from build123d import *

# Parameters (mm, degrees)
BOSS_EXTRUDE1_DEPTH = 155.575
SKETCH3_R           = 2.6289
CUT_EXTRUDE2_DEPTH  = 25.4
SKETCH4_R           = 2.6289
CUT_EXTRUDE3_DEPTH  = 25.4


with BuildPart() as part:
    # Sketch1 → Boss-Extrude1 (new body)
    with BuildSketch(Plane.XY):
        Polygon((3.484491601, 6.45148445), (-3.844903625, 6.243400471), (-7.329395227, -0.208083979), (-3.484491601, -6.45148445), (3.844903625, -6.243400471), (7.329395227, 0.208083979), align=None)
    extrude(amount=BOSS_EXTRUDE1_DEPTH)

    # Sketch3 → Cut-Extrude2 (cut)
    with BuildSketch(Plane.XY.offset(155.575)):
        Circle(SKETCH3_R)
    extrude(amount=-CUT_EXTRUDE2_DEPTH, mode=Mode.SUBTRACT)

    # Sketch4 → Cut-Extrude3 (cut)
    with BuildSketch(Plane(origin=(0, 0, 0), x_dir=(-1, 0, 0), z_dir=(0, 0, -1))):
        Circle(SKETCH4_R)
    extrude(amount=-CUT_EXTRUDE3_DEPTH, mode=Mode.SUBTRACT)


solid = part.part
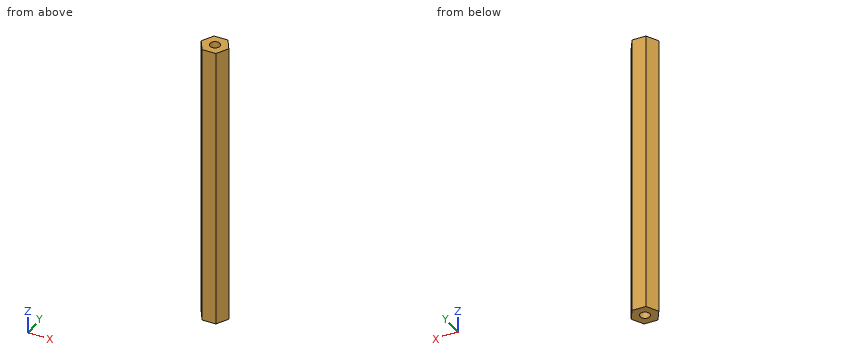
Geometry check sheet. Reference: the model listing, model coordinates, mm. Give positions to 0.01 mm unless a question says otherwise; leave off trailing zeros. Order: outer loops, then holes, each group sorted by start corner. A loop starts at its lowest first (then second) coordinate and runs counter-clockwise, first axis right, second up. Notation, with made-up numbers: M 4,53 L 26,53 A30 cw 26,77 Z; hole C -12,16 d1. An arc over 180 degrees is marked long. Use a Markdown table: item, result.
Item 1: Section check C-C (x = -0.5). Record the cut outline in (y, z) (3 decimals).
Answers follow:
| item | result |
|---|---|
| outline | M -6.367,0 L -2.581,0 L -2.581,25.4 L 2.581,25.4 L 2.581,0 L 6.338,0 L 6.338,155.575 L 2.581,155.575 L 2.581,130.175 L -2.581,130.175 L -2.581,155.575 L -6.367,155.575 Z |
Item 2: Section check B-B (z = 60.5). Record the cut outline in (x, y), and give its area (3 significant figures).
Answers follow:
| item | result |
|---|---|
| outline | M -7.33,-0.21 L -3.48,-6.45 L 3.84,-6.24 L 7.33,0.21 L 3.48,6.45 L -3.84,6.24 Z |
| area | 140 mm2 |
Item 3: Section check D-D (y = -4). Record the cut outline in (x, z) (3 decimals).
Answers follow:
| item | result |
|---|---|
| outline | M -4.994,0 L 5.057,0 L 5.057,155.575 L -4.994,155.575 Z |
Item 4: Section check A-A (z = 22). Record the cut outline in (x, y).
Answers follow:
| item | result |
|---|---|
| outline | M -7.33,-0.21 L -3.48,-6.45 L 3.84,-6.24 L 7.33,0.21 L 3.48,6.45 L -3.84,6.24 Z; hole C 0,0 d5.26 |
Item 5: Depth check by flat-ended pin: P1, Ø4, axis at x = -0.5, y = 1, coming from the -Z side; P2, Ø2, axis at x = 1, z = 82.5, coming from the +Y side; P3, Ø5, axis at y = -4, z = 25.5, coming from the -X side; P4, Ø2.5, axis at x = -1, y = -0.5, coming from the +Z side (3 decimals). Enter the tip coordinate at first touch or a pass-through.
Answers follow:
| item | result |
|---|---|
| P1 | stops at z = 0 |
| P2 | stops at y = 6.41 |
| P3 | stops at x = -6.53 |
| P4 | stops at z = 130.175 |
Item 6: Material ranges on line 1 along Z through (x, y) = (-0.25, 2) (3 decimals); line 2 along Y through (x, z) = (0, 15); line 3 along Y through (x, z) = (-0.75, 15), recorded low to high.
Answers follow:
| item | result |
|---|---|
| line 1 | z = 25.4 to 130.175 |
| line 2 | y = -6.35 to -2.63, 2.63 to 6.35 |
| line 3 | y = -6.37 to -2.52, 2.52 to 6.33 |
